Build history of the part. All positions in model axes, mm. A direction names the side the tool comes from. Give positions to 0.01 mm unless a question says otherwise; leave off trailing zeros. Order: outer loops, then holes, each group sorted by start corner. A loop starts at its lowest first (then second) coordinate and runs counter-clockwise, first axis right, second up. Notation, with made-up numbers: M -32,-34.5 L -7,-34.5 A12 ccw -7,-17.5 Z; hole C 88.25,32.25 d6. An arc over 180 degrees is marked long. One line per item, written item: value.
from build123d import *

# Parameters (mm, degrees)
FILLET1_R          = 0.2
SKETCH1_R          = 2.974873734
CUT_EXTRUDE1_DEPTH = 0.45


# Read off the part's stored shape, not the designer's step: Stock-Finger_Rubber_Sensor+Button-1
with BuildPart() as part:
    # Stock-Finger_Rubber_Sensor+Button-1 outl → Stock-Finger_Rubber_Sensor+Button-1 (revolve)
    with BuildSketch(Plane.XY.offset(29.325)):
        with BuildLine():
            Line((1.9, 3.4), (1.9, -0.158502039))
            Line((1.9, -0.158502039), (1.5, -0.158502039))
            Line((1.5, -0.158502039), (1.5, 2.5))
            Line((1.5, 2.5), (0, 2.5))
            Line((0, 2.5), (0, -1.498502039))
            Line((0, -1.498502039), (2.3, -1.498502039))
            ThreePointArc((2.3, -1.498502039), (2.370710678, -1.469212717), (2.4, -1.398502039))
            Line((2.4, -1.398502039), (2.4, 2.4))
            Line((2.4, 2.4), (3.4, 2.4))
            Line((3.4, 2.4), (3.4, 3.4))
            Line((3.4, 3.4), (1.9, 3.4))
        make_face()
    revolve(axis=Axis((0, 0, 29.325), (0, 1, 0)))

    # Fillet1
    fillet1_edges = [part.edges().sort_by_distance(p)[0] for p in [
        (-3.4, 2.4, 29.325),
    ]]
    fillet(fillet1_edges, radius=FILLET1_R)

    # Sketch1 → Cut-Extrude1 (cut)
    with BuildSketch(Plane(origin=(0, 3.4, 0), x_dir=(1, 0, 0), z_dir=(0, 1, 0))):
        with Locations(Location((0, -29.325, 0), (0, 0, 270))):
            Circle(SKETCH1_R)
    extrude(amount=-CUT_EXTRUDE1_DEPTH, mode=Mode.SUBTRACT)


solid = part.part
1) Saw through at C-C, the plane y = -0.4. Write the cut outline in (x, z) (3 decimals), then the cut area to 3 significant figures.
Check values:
outline: C 0,29.325 d4.8
area: 18.1 mm^2
2) Saw through at B-B, the plane y = 1.3. Write the cut outline in (x, z) (3 decimals), then the cut area to 3 significant figures.
Check values:
outline: C 0,29.325 d4.8; C 0,29.325 d3; hole C 0,29.325 d3.8
area: 13.8 mm^2
3) Pin check, flat tips, straight feed: pin 1 (1.8 mm diameter, centred on x = -0.5, z = 30.5, fed in from +Y); pin 2 (1.5 mm diameter, centred on x = 0.5, y = 0.5, fed in from -Z) (3 decimals); pin 3 (2 mm diameter, centred on y = 0.5, z = 30.5, fed in from -X). Stop position of each tip, or through.
Check values:
pin 1: y = 2.95
pin 2: z = 26.925
pin 3: x = -2.39
4) Mould opens along X. For faces 3 (the face through (-0.312, 0.527, 26.945)), 4 (the face through (0, -1.499, 29)), 5 (the face through (-0.2, 1.19, 27.84)) say: released by +X, released by -X, zero draft, split by the parting line, or undercut.
Check values:
face 3: split by the parting line
face 4: zero draft
face 5: undercut
5) Drill centre lines: probe 1 along Z at (x, y) = (0, 0.5) (3 decimals); probe 2 along Z at (x, y) = (-0.75, 1); probe 3 along Y at (x, z) = (-1.25, 30). Where is each one in solid material? Low to high. Write a range as from..to.
Check values:
probe 1: 26.925..27.425, 27.825..30.825, 31.225..31.725
probe 2: 27.05..27.58, 28.03..30.62, 31.07..31.6
probe 3: -1.5..2.5
6) Tool access for faces 1 (the face through (-0.443, 3.006, 25.954)), 2 (the face through (-0.6, 2.95, 31.3)): list every direction of +Z, -Z, +X, -X, +Y, -Y with a clear straight run to the whole face (end or side of a thin tool).
Check values:
face 1: +Y, -Y
face 2: +Y
